```python
from build123d import *

# Parameters (mm, degrees)
SKETCH1_W               = 200
SKETCH1_H               = 200
BOSS_EXTRUDE1_DEPTH     = 300
SKETCH2_R               = 75
CUT_EXTRUDE1_DEPTH      = 50
CUT_EXTRUDE2_DEPTH      = 201
FILLET1_R               = 30
FILLET2_R               = 20
SKETCH4_W               = 200
SKETCH4_H               = 120
CUT_EXTRUDE3_DEPTH      = 149
SKETCH7_R               = 15
CUT_EXTRUDE4_DEPTH      = 200
CUT_EXTRUDE4_DEPTH_BACK = 149
SKETCH8_W               = 150
SKETCH8_H               = 50
BOSS_EXTRUDE2_DEPTH     = 10
FILLET3_R               = 7
SKETCH9_W               = 150
SKETCH9_H               = 50
BOSS_EXTRUDE3_DEPTH     = 10
FILLET4_R               = 7


with BuildPart() as part:
    # Sketch1 → Boss-Extrude1 (new body)
    with BuildSketch(Plane(origin=(0, 0, 0), x_dir=(1, 0, 0), z_dir=(0, 1, 0))):
        Rectangle(SKETCH1_W, SKETCH1_H)
    extrude(amount=BOSS_EXTRUDE1_DEPTH)

    # Sketch2 → Cut-Extrude1 (cut)
    with BuildSketch(Plane.XZ):
        Circle(SKETCH2_R)
    extrude(amount=-CUT_EXTRUDE1_DEPTH, mode=Mode.SUBTRACT)

    # Sketch3 → Cut-Extrude2 (cut, through all)
    with BuildSketch(Plane.XY.offset(100)):
        Polygon((-100, 95.980685294), (-19.135993401, 213.188644877), (100, 75.250025776), (100, 300), (-100, 300), align=None)
    extrude(amount=-CUT_EXTRUDE2_DEPTH, mode=Mode.SUBTRACT)

    # Fillet1
    fillet1_edges = [part.edges().sort_by_distance(p)[0] for p in [
        (-19.135993401, 213.188644877, 0),
    ]]
    fillet(fillet1_edges, radius=FILLET1_R)

    # Fillet2
    fillet2_edges = [part.edges().sort_by_distance(p)[0] for p in [
        (-100, 95.980685294, 0),
        (100, 75.250025776, 0),
    ]]
    fillet(fillet2_edges, radius=FILLET2_R)

    # Sketch4 → Cut-Extrude3 (cut)
    with BuildSketch(Plane(origin=(0, 200, 0), x_dir=(1, 0, 0), z_dir=(0, 1, 0))):
        Rectangle(SKETCH4_W, SKETCH4_H)
    extrude(amount=-CUT_EXTRUDE3_DEPTH, mode=Mode.SUBTRACT)

    # Sketch7 → Cut-Extrude4 (cut, two sides)
    with BuildSketch(Plane(origin=(0, 0, 60), x_dir=(-1, 0, 0), z_dir=(0, 0, -1))) as cut_extrude4_sk:
        with Locations((20, 170.784862367)):
            Circle(SKETCH7_R)
    extrude(amount=CUT_EXTRUDE4_DEPTH, mode=Mode.SUBTRACT)
    extrude(cut_extrude4_sk.sketch, amount=-CUT_EXTRUDE4_DEPTH_BACK, mode=Mode.SUBTRACT)

    # Sketch8 → Boss-Extrude2 (add)
    with BuildSketch(Plane.XY.offset(100)):
        with Locations((0, 35.260136057)):
            Rectangle(SKETCH8_W, SKETCH8_H)
    extrude(amount=BOSS_EXTRUDE2_DEPTH)

    # Fillet3
    fillet3_edges = [part.edges().sort_by_distance(p)[0] for p in [
        (-75, 35.260136057, 110),
        (0, 10.260136057, 110),
        (75, 35.260136057, 110),
        (0, 60.260136057, 110),
    ]]
    fillet(fillet3_edges, radius=FILLET3_R)

    # Sketch9 → Boss-Extrude3 (add)
    with BuildSketch(Plane(origin=(0, 0, -100), x_dir=(-1, 0, 0), z_dir=(0, 0, -1))):
        with Locations((0, 35.002047413)):
            Rectangle(SKETCH9_W, SKETCH9_H)
    extrude(amount=BOSS_EXTRUDE3_DEPTH)

    # Fillet4
    fillet4_edges = [part.edges().sort_by_distance(p)[0] for p in [
        (75, 35.002047413, -110),
        (0, 10.002047413, -110),
        (-75, 35.002047413, -110),
        (0, 60.002047413, -110),
    ]]
    fillet(fillet4_edges, radius=FILLET4_R)


solid = part.part
```
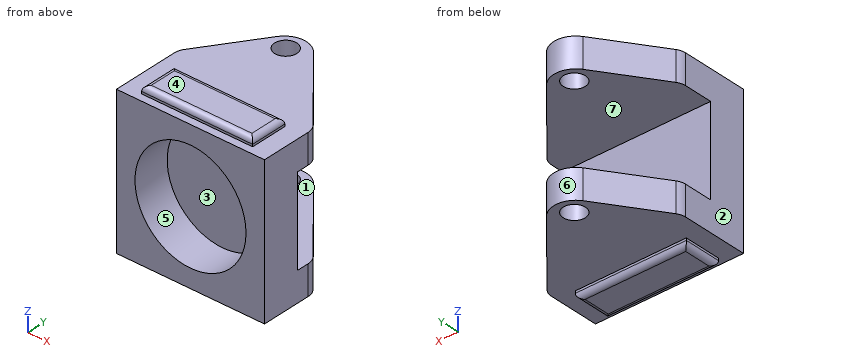
For this review, take the finished solid that the model builds, in its own axes (mm). Face numbers are marked on the shaded views. A direction names the side the tool comes from. Round coordinates to 2 decimals unless told otherwise and drop trailing zeros. Loops run counter-clockwise (first coordinate to the right, second up) from the corner with the lowest first, then second, coordinate; pieces in that order, holes last.
Q1. Add section A-A on y = 96. Write out the cut boundary in (x, z).
Result sheet:
outline: (-99, -100) - (82.08, -100) - (82.08, -60) - (-99, -60) - close; (-99, 60) - (82.08, 60) - (82.08, 100) - (-99, 100) - close
Q2. Add section D-D on z = -84.5. Write out the cut boundary in (x, y), plus the area to 3 significant figures.
Result sheet:
outline: (-100, 0) - (100, 0) - (100, 67.81) arc R20 ccw to (95.14, 80.88) - (6.23, 183.82) arc R30 ccw to (-41.17, 181.25) - (-96.46, 101.11) arc R20 ccw to (-100, 89.75) - close; hole circle Ø30 at (-20, 170.78)
area: 28,600 mm2
Q3. Mouldability with a two-part tool opening along Z and no side actions: class the marked faces 1, 2, 3 and 4 as +Z half, -Z half, draft (parallel to the pull), parting line (faces both ways), or undercut.
Result sheet:
face 1: undercut
face 2: draft
face 3: undercut
face 4: +Z half
Q4. Insertion check: pin 1 Ø0.9 at (y, z) = (41.5, 101.5) entering from -X; pin 2 Ø5 at (y, z) = (85, 85) entering from +X; pin 3 Ø0.9 at (y, z) = (26.5, 102) entering from +X; pin 4 Ø18 at (x, y) = (-20, 170.78) entering from -Z. Each pin has a flat end and moves straight along its axis. Give the tip position at first contact, or say it passes through.
Result sheet:
pin 1: stops at x = -75
pin 2: stops at x = 93.74
pin 3: stops at x = 75
pin 4: passes through
Q5. Machinability: for the marked faces 5, 6 and 7, which of the approach directions +Z, -Z, +X, -X, +Y, -Y give a long, thin tool a straight path to every point of the face, cutting with its end or side? Answer none if there is none.
Result sheet:
face 5: -Y
face 6: +Z, -Z, +Y
face 7: +X, -X, +Y
Q6. To check wall thickness, follow line 1 along Z through (x, y) = (0, 33); line 2 along Z through (x, y) = (61, 116); line 3 along Y through (x, z) = (-19.5, -42). State the ranges of each line that lie inside material, in increasing order.
Result sheet:
line 1: z = -110 to -75, 75 to 110
line 2: z = -100 to -60, 60 to 100
line 3: y = 50 to 51
Q7. Add section C-C on x = -20. Give the number of separate pieces and of enclosed holes in the cut face, plus the area to 3 significant figures.
Result sheet:
separate pieces: 3
enclosed holes: 0
area: 13,000 mm2
Q8. Add section B-B on z = 0. Write out the cut boundary in (x, y).
Result sheet:
outline: (-100, 0) - (-75, 0) - (-75, 50) - (75, 50) - (75, 0) - (100, 0) - (100, 51) - (-100, 51) - close
